The model under review builds one solid part; all positions refer to its coordinate system, in mm. Coordinates: 2 decimals unless noted, no trailing zeros. Loops run counter-clockwise (first coordinate to the right, second up) from the corner with the lowest first, then second, coordinate; pieces in that order, holes last. Notation, with made-up numbers: M -34,16 L -3,16 A12 cw -3,32 Z; hole C 10.25,-11.75 d11. An arc over 180 degrees is marked long. Use CSV: the item, a comma, the result in double quotes. Start each with the question number.
from build123d import *

# Parameters (mm, degrees)
BOSS_EXTRUDE1_DEPTH = 0.254
SKETCH2_R           = 4.699
CUT_EXTRUDE1_DEPTH  = 1.254
SKETCH3_W           = 2.54
SKETCH3_H           = 0.635
CUT_EXTRUDE2_DEPTH  = 1.254
CUT_EXTRUDE4_DEPTH  = 1.254
CUT_EXTRUDE5_DEPTH  = 1.254


with BuildPart() as part:
    # Sketch1 → Boss-Extrude1 (new body)
    with BuildSketch(Plane.XY):
        with BuildLine():
            Line((67.21146711, 76.191723231), (8.696654013, 17.676910134))
            Line((8.696654013, 17.676910134), (7.228954972, 14.133571205))
            ThreePointArc((7.228954972, 14.133571205), (14.666587579, 6.075099489), (15.105587123, -4.88230096))
            Line((15.105587123, -4.88230096), (18.648926052, -6.35))
            Line((18.648926052, -6.35), (101.401368334, -6.35))
            ThreePointArc((101.401368334, -6.35), (93.866160503, 38.880636728), (67.21146711, 76.191723231))
        make_face()
        with BuildLine():
            Line((88.672924278, 6.35), (27.86051193, 6.35))
            ThreePointArc((27.86051193, 6.35), (26.399857642, 10.93517908), (24.190484974, 15.210228852))
            Line((24.190484974, 15.210228852), (67.191354125, 58.211098004))
            ThreePointArc((67.191354125, 58.211098004), (82.13289044, 34.020557137), (88.672924278, 6.35))
        make_face(mode=Mode.SUBTRACT)
    extrude(amount=BOSS_EXTRUDE1_DEPTH)

    # Sketch2 → Cut-Extrude1 (cut, through all)
    with BuildSketch(Plane.XY.offset(0.254)):
        with Locations((22.225, 0)):
            Circle(SKETCH2_R)
        with Locations((36.195, 0)):
            Circle(SKETCH2_R)
        with Locations((61.722, 0)):
            Circle(SKETCH2_R)
        with Locations((75.692, 0)):
            Circle(SKETCH2_R)
        with Locations((95.25, 0)):
            Circle(SKETCH2_R)
        with Locations((15.715448212, 15.715448212)):
            Circle(SKETCH2_R)
        with Locations((25.593729945, 25.593729945)):
            Circle(SKETCH2_R)
        with Locations((43.644044748, 43.644044748)):
            Circle(SKETCH2_R)
        with Locations((53.522326482, 53.522326482)):
            Circle(SKETCH2_R)
        with Locations((92.004434954, 24.652514046)):
            Circle(SKETCH2_R)
        with Locations((82.48891971, 47.625)):
            Circle(SKETCH2_R)
        with Locations((67.351920908, 67.351920908)):
            Circle(SKETCH2_R)
    extrude(amount=-CUT_EXTRUDE1_DEPTH, mode=Mode.SUBTRACT)

    # Sketch3 → Cut-Extrude2 (cut, through all)
    with BuildSketch(Plane.XY.offset(0.254)):
        Polygon((15.266435406, 24.246691527), (17.06248663, 26.042742751), (17.511499436, 25.593729945), (15.715448212, 23.797678721), align=None)
        Polygon((44.991083167, 53.971339288), (43.195031942, 52.175288063), (43.644044748, 51.726275257), (45.440095973, 53.522326482), align=None)
        with Locations((29.21, -6.0325)):
            Rectangle(SKETCH3_W, SKETCH3_H)
        with Locations((68.707, -6.0325)):
            Rectangle(SKETCH3_W, SKETCH3_H)
        Polygon((29.230733674, 38.210989795), (31.026784898, 40.007041019), (31.475797704, 39.558028213), (29.67974648, 37.761976989), align=None)
        Polygon((56.845021246, 65.825277367), (55.048970022, 64.029226143), (55.497982828, 63.580213337), (57.294034052, 65.376264561), align=None)
        with Locations((48.9585, -6.0325)):
            Rectangle(SKETCH3_W, SKETCH3_H)
        with Locations((85.471, -6.0325)):
            Rectangle(SKETCH3_W, SKETCH3_H)
        Polygon((99.935462164, 14.437711971), (100.266998693, 11.919442024), (101.526133667, 12.085210288), (101.194597138, 14.603480236), align=None)
        Polygon((93.765504959, 37.464305742), (94.938831965, 37.950313702), (93.966816047, 40.296967714), (92.793489041, 39.810959755), align=None)
        Polygon((79.327792988, 62.471156422), (80.874047017, 60.456038938), (81.88160576, 61.229165953), (80.33535173, 63.244283437), align=None)
        Polygon((13.593916116, 7.005422516), (14.565932035, 4.658768503), (15.739259041, 5.144776462), (14.767243123, 7.491430475), align=None)
    extrude(amount=-CUT_EXTRUDE2_DEPTH, mode=Mode.SUBTRACT)

    # Sketch6 → Cut-Extrude4 (cut, through all)
    with BuildSketch(Plane.XY.offset(0.254)):
        with BuildLine():
            Line((12.392753447, 19.038142977), (22.27103518, 28.91642471))
            ThreePointArc((22.27103518, 28.91642471), (28.91642471, 28.91642471), (28.91642471, 22.27103518))
            Line((28.91642471, 22.27103518), (19.038142977, 12.392753447))
            ThreePointArc((19.038142977, 12.392753447), (12.392753447, 12.392753447), (12.392753447, 19.038142977))
        make_face()
        with BuildLine():
            Line((40.321349984, 46.966739513), (50.199631717, 56.845021246))
            ThreePointArc((50.199631717, 56.845021246), (56.845021246, 56.845021246), (56.845021246, 50.199631717))
            Line((56.845021246, 50.199631717), (46.966739513, 40.321349984))
            ThreePointArc((46.966739513, 40.321349984), (40.321349984, 40.321349984), (40.321349984, 46.966739513))
        make_face()
        with BuildLine():
            Line((22.225, 4.699), (36.195, 4.699))
            ThreePointArc((36.195, 4.699), (40.894, 0), (36.195, -4.699))
            Line((36.195, -4.699), (22.225, -4.699))
            ThreePointArc((22.225, -4.699), (17.526, 0), (22.225, 4.699))
        make_face()
        with BuildLine():
            Line((61.722, 4.699), (75.692, 4.699))
            ThreePointArc((75.692, 4.699), (80.391, 0), (75.692, -4.699))
            Line((75.692, -4.699), (61.722, -4.699))
            ThreePointArc((61.722, -4.699), (57.023, 0), (61.722, 4.699))
        make_face()
        with BuildLine():
            ThreePointArc((86.558373083, 49.9745), (79.294873009, 60.845096068), (70.674615673, 70.674615673))
            ThreePointArc((70.674615673, 70.674615673), (64.029226143, 70.674615673), (64.029226143, 64.029226143))
            ThreePointArc((64.029226143, 64.029226143), (71.838938317, 55.123956158), (78.419466338, 45.2755))
            ThreePointArc((78.419466338, 45.2755), (84.83841971, 43.555546628), (86.558373083, 49.9745))
        make_face()
    extrude(amount=-CUT_EXTRUDE4_DEPTH, mode=Mode.SUBTRACT)

    # Sketch5 → Cut-Extrude5 (cut, through all)
    with BuildSketch(Plane.XY.offset(0.254)):
        Polygon((86.614, -7.62), (86.614, 10.250086524), (102.87, 12.390229525), (102.87, -7.62), align=None)
    extrude(amount=-CUT_EXTRUDE5_DEPTH, mode=Mode.SUBTRACT)


solid = part.part
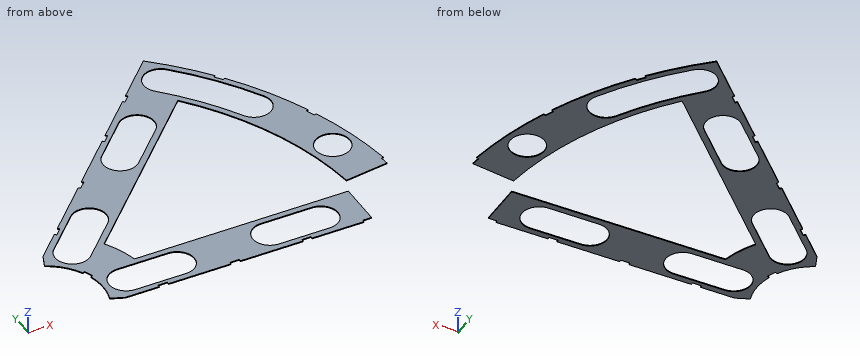
1. Insertion check: pin 1 Ø15 at (x, y) = (92, 24.65) entering from -Z. The pin has a flat end and moves straight along its axis. Give the tip position at first contact, or say it passes through.
2. To check wall thickness, follow line 1 along X through (y, z) = (0, 0.1) (3 decimals); line 2 along Y through (x, z) = (77, 0.1); line 3 along Y through (x, z) = (63.5, 0.15). State the ranges of each line that lie inside material, in increasing order.
3. Add section A-A (y = 0). Write out the cut boundary in (x, z) (3 decimals).
4. Add section B-B (y = 32). Write out the cut boundary in (x, z).
5. Add section C-C (z = 0.15). Give the number of separate pieces and of enclosed holes in the cut face, plus the area to 3 significant figures.
Solved:
1,pin 1,"stops at z = 0"
2,line 1,"x = 15.875 to 17.526, 40.894 to 57.023, 80.391 to 86.614"
2,line 2,"y = -6.35 to -4.51, 4.51 to 6.35, 44.43 to 47.65, 63.72 to 66.28"
2,line 3,"y = -6.35 to -4.7, 4.7 to 6.35, 54.52 to 64.66, 70.04 to 72.48"
3,outline,"M 15.875,0 L 17.526,0 L 17.526,0.254 L 15.875,0.254 Z; M 40.894,0 L 57.023,0 L 57.023,0.254 L 40.894,0.254 Z; M 80.391,0 L 86.614,0 L 86.614,0.254 L 80.391,0.254 Z"
4,outline,"M 23.02,0 L 40.98,0 L 40.98,0.25 L 23.02,0.25 Z; M 82.94,0 L 96.43,0 L 96.43,0.25 L 82.94,0.25 Z"
5,separate pieces,"1"
5,enclosed holes,"6"
5,area,"1,580 mm^2"
